```python
from build123d import *

# Parameters (mm, degrees)
SKETCH_W     = 70
SKETCH_H     = 80
PAD_DEPTH    = 3
SKETCH001_R  = 1.5
PAD001_DEPTH = 40
SKETCH002_R  = 1.5
POCKET_DEPTH = 77.001


with BuildPart() as part:
    # Sketch → Pad (new body)
    with BuildSketch(Plane.XY):
        with Locations((0, 40)):
            Rectangle(SKETCH_W, SKETCH_H)
    extrude(amount=PAD_DEPTH)

    # Sketch001 (on Face6 of Pad) → Pad001 (join)
    with BuildSketch(Plane.XY.offset(3)):
        Polygon((-35, 0), (-35, 80), (-32, 80), (-32, 77), (-22, 77), (-22, 67), (-32, 67), (-32, 13), (-22, 13), (-22, 3), (-32, 3), (-32, 0), align=None)
        with Locations((-27, 8)):
            Circle(SKETCH001_R, mode=Mode.SUBTRACT)
        with Locations((-27, 72)):
            Circle(SKETCH001_R, mode=Mode.SUBTRACT)
        Polygon((35, 80), (35, 0), (32, 0), (32, 3), (22, 3), (22, 13), (32, 13), (32, 67), (22, 67), (22, 77), (32, 77), (32, 80), align=None)
        with Locations((27, 8)):
            Circle(SKETCH001_R, mode=Mode.SUBTRACT)
        with Locations((27, 72)):
            Circle(SKETCH001_R, mode=Mode.SUBTRACT)
    extrude(amount=PAD001_DEPTH)

    # Sketch002 (on Face21 of Pad001) → Pocket (cut, through all)
    with BuildSketch(Plane.XZ.offset(-3)):
        with Locations((27, 23)):
            Circle(SKETCH002_R)
        with Locations((-27, 23)):
            Circle(SKETCH002_R)
    extrude(amount=-POCKET_DEPTH, mode=Mode.SUBTRACT)


solid = part.part
```
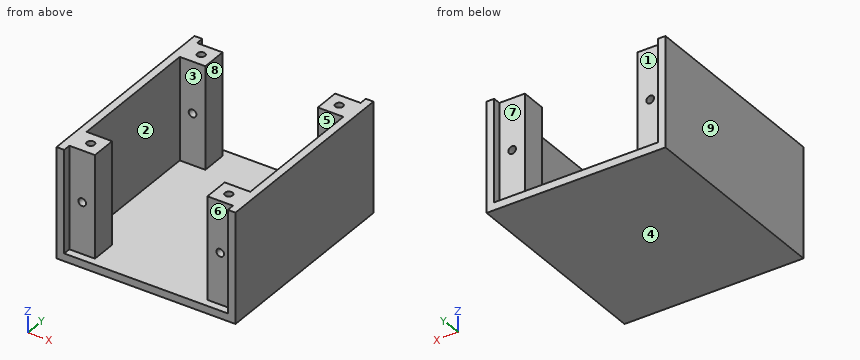
Geometry: final body of the model. Coordinates: model frame, mm. Face numbers are marked on the shaded views. A direction names the side the tool comes from. Coordinates: 2 decimals unless noted, no trailing zeros. Order: outer loops, then holes, each group sorted by start corner. A loop starts at its lowest first (then second) coordinate and runs counter-clockwise, first axis right, second up. Notation, with made-up numbers: (-16, 61) - (-8, 61) arc R22 cw to (-8, 89) - close; hole circle Ø10 at (-29.5, 3.25). An arc over 180 degrees is marked (long way). Return JSON: item names as keys, results as strings. Group by question number.
1. Cut plane B-B (x = 30.5). Output: boundary loops of the cut face in (y, z), plus the area to 3 significant figures.
2. Pin query (flat end, axial travel): pin 1 (1.5 mm diameter, centred on x = 27, y = 7.5, fed in from +Z); pin 2 (3 mm diameter, centred on x = -29.5, z = 29.5, fed in from +Y); pin 3 (4 mm diameter, centred on x = -27, z = 23, fed in from -Y); pin 4 (1.5 mm diameter, centred on x = -9, z = 5.5, fed in from +Y). Return the tip coordinate at first contact, or that it passes through.
3. Cut plane A-A (z = 17). Output: boundary loops of the cut face in (x, y), plus the area to 3 significant figures.
4. Set-up query: the marked faces 5, 6, 7, 8 and 9. Return all of +Z, -Z, +X, -X, +Y, -Y with unobstructed straight access to the full face (end or side cutting, diameter ignored); none if empty.
5. Cut plane C-C (x = 18). Output: boundary loops of the cut face in (y, z), plus the area to 3 significant figures.
6. Material intervals for line 1 along X through (y, z) = (8, 37); line 2 along Y through (x, z) = (-27, 13.5); line 3 along X through (y, z) = (50.5, 29.5), sorted ascending. Write a range as [from, to].
7. Pull-direction query (Y, two-part tool) for the marked faces 1, 2, 3 and 4; classes: pulls with the +Y half, pulls with the -Y half, needs draft (parallel to the pull), parting line crosses it, or undercut.
Resolved:
{
 "1": {"outline": "(0, 0) - (80, 0) - (80, 3) - (77, 3) - (77, 43) - (67, 43) - (67, 3) - (13, 3) - (13, 43) - (3, 43) - (3, 3) - (0, 3) - close", "area": "1,040 mm²"},
 "2": {"pin 1": "stops at z = 3", "pin 2": "stops at y = 77", "pin 3": "stops at y = 3", "pin 4": "passes through"},
 "3": {"outline": "(-35, 0) - (-32, 0) - (-32, 3) - (-22, 3) - (-22, 13) - (-32, 13) - (-32, 67) - (-22, 67) - (-22, 77) - (-32, 77) - (-32, 80) - (-35, 80) - close; (22, 3) - (32, 3) - (32, 0) - (35, 0) - (35, 80) - (32, 80) - (32, 77) - (22, 77) - (22, 67) - (32, 67) - (32, 13) - (22, 13) - close; hole circle Ø3 at (-27, 8); hole circle Ø3 at (-27, 72); hole circle Ø3 at (27, 8); hole circle Ø3 at (27, 72)", "area": "852 mm²"},
 "4": {"face 5": "+Z", "face 6": "+Z, -Y", "face 7": "+Z, +Y", "face 8": "+Z, +Y, -Y", "face 9": "+Z, -Z, -X, +Y, -Y"},
 "5": {"outline": "(0, 0) - (80, 0) - (80, 3) - (0, 3) - close", "area": "240 mm²"},
 "6": {"line 1": "x = [-35, -28.5], [-25.5, -22], [22, 25.5], [28.5, 35]", "line 2": "y = [3, 6.5], [9.5, 13], [67, 70.5], [73.5, 77]", "line 3": "x = [-35, -32], [32, 35]"},
 "7": {"face 1": "pulls with the +Y half", "face 2": "undercut", "face 3": "undercut", "face 4": "needs draft"}
}
